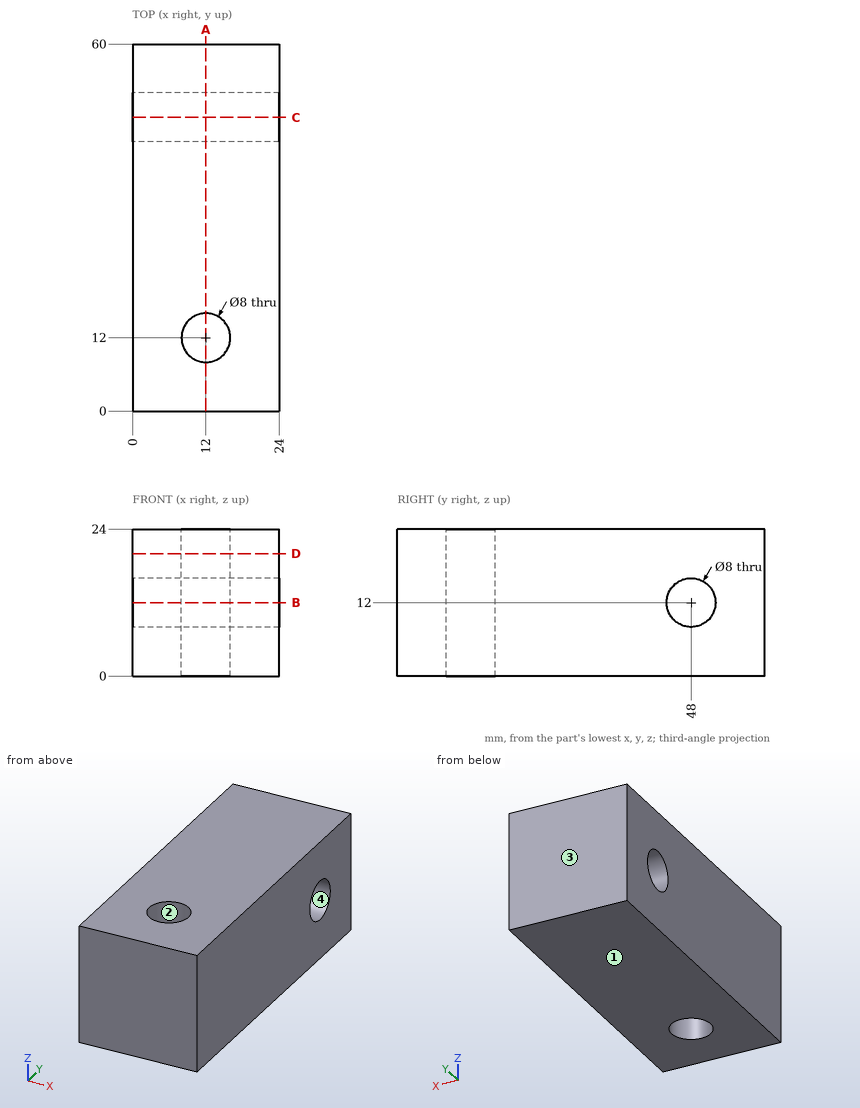
Design review of the part shown in the three views and the two pictorial views. Dimensions are in mm from the part's minimum x, y and z. Round coordinates to 2 decimals unless told otherwise and drop trailing zeros. Loops run counter-clockwise (first coordinate to the right, second up) from the corner with the lowest first, then second, coordinate; pieces in that order, holes last. Notation, with made-up numbers: M 65.25,79.5 L 120.25,79.5 A18 cw 120.25,113.5 Z; hole C 3.5,63.5 d5. An arc over 180 degrees is marked long. Answer as a JSON object with one key per item and string values.
Item 1: We need section D-D on z = 20. Give the boundary of the cut face in (x, y), and give its area (3 significant figures).
Answer sheet:
{"outline": "M 0,0 L 24,0 L 24,60 L 0,60 Z; hole C 12,12 d8", "area": "1,390 mm^2"}
Item 2: Wall thickness on L1, parallel to Z at x = 16, y = 48; L2, parallel to Y at x = 12, z = 7: over which ranges is each line inside the solid? List them lowest first. Write a range as from..to.
Answer sheet:
{"L1": "z = 0..8, 16..24", "L2": "y = 0..8, 16..60"}
Item 3: The part is to be moulded in two halves that separate along Y. For the marked faces 1, 2, 3 and 4, say which applies: pulls with the +Y half, pulls with the -Y half, needs draft (parallel to the pull), parting line crosses it, or undercut.
Answer sheet:
{"face 1": "needs draft", "face 2": "undercut", "face 3": "pulls with the +Y half", "face 4": "undercut"}
Item 4: We need section A-A on x = 12. Give the boundary of the cut face in (y, z), and give its area (3 significant figures).
Answer sheet:
{"outline": "M 0,0 L 8,0 L 8,24 L 0,24 Z; M 16,0 L 60,0 L 60,24 L 16,24 Z; hole C 48,12 d8", "area": "1,200 mm^2"}
Item 5: We need section B-B on z = 12. Give the boundary of the cut face in (x, y).
Answer sheet:
{"outline": "M 0,0 L 24,0 L 24,44 L 0,44 Z; M 0,52 L 24,52 L 24,60 L 0,60 Z; hole C 12,12 d8"}
Item 6: We need section C-C on y = 48. Give the boundary of the cut face in (x, z), and give its area (3 significant figures).
Answer sheet:
{"outline": "M 0,0 L 24,0 L 24,8 L 0,8 Z; M 0,16 L 24,16 L 24,24 L 0,24 Z", "area": "384 mm^2"}
